Part print with two shaded views. Sizes in mm from the minimum x, y, z corner. A direction names the side the tool comes from. Give positions to 0.01 mm unless a question says otherwise; leave off trailing zeros. Write each loop counter-clockwise with the first axis right and the second up, starting at its lowest first coordinate (ties: lowest second). Pieces come first, ordered by that corner, then holes. Notation, with made-up numbers: (-20, 23.25) -> (11, 23.25) arc R25 ccw to (11, 60.25) -> close; hole circle Ø5 at (-11, -7.5). An arc over 180 degrees is marked (long way). Answer in a Markdown table with one row per item. Add a question column.
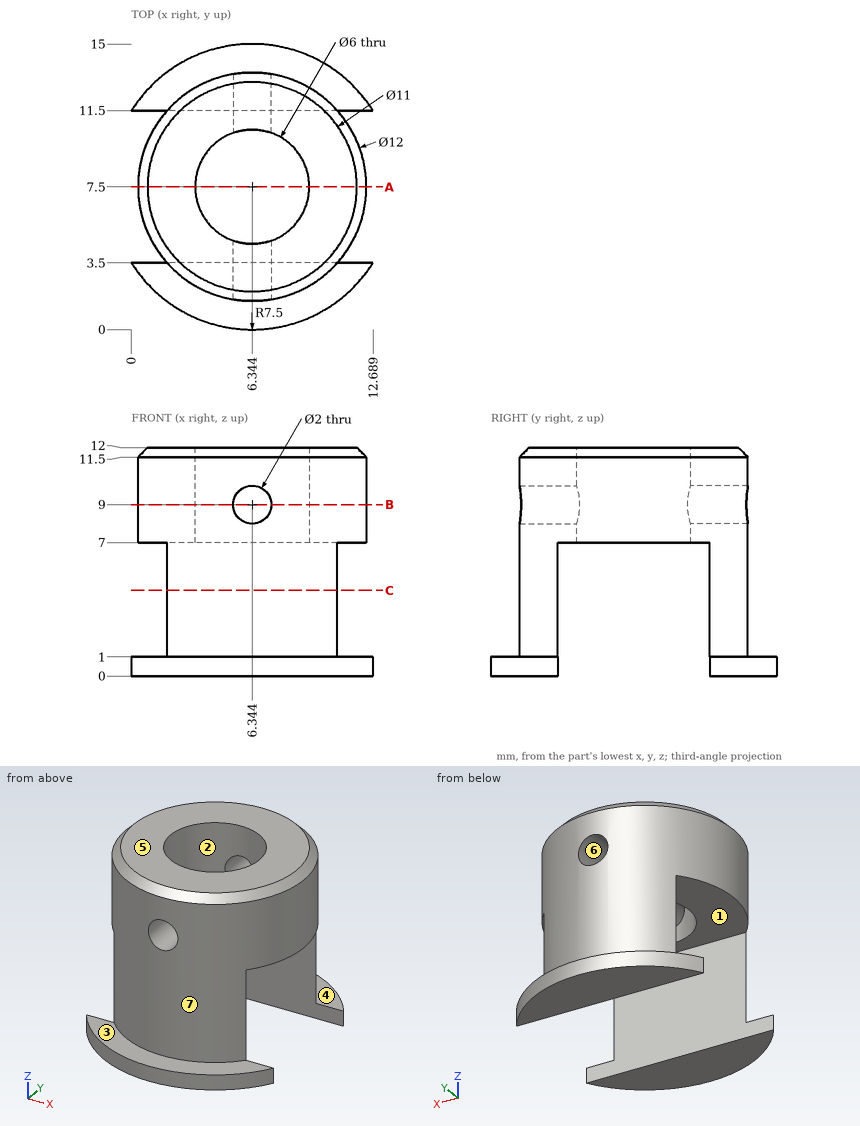
Item 1: Slice it at B-B, the plane z = 9. List the corners of the cut face in (x, y) (1 decimal).
Item 2: Slice it at C-C, the plane z = 4.5. List the corners of the cut face in (x, y) (1 decimal).
Item 3: Drop flat-ended pins along their axis: pin 1 Ø3 at (x, y) = (2, 12.5) entering from -Z; pin 2 Ø3 at (x, z) = (9, 3) entering from +Y; pin 3 Ø2 at (x, z) = (6.5, 4.5) entering from -Y. Give the stop position or say it passes through.
Item 4: Mould opens along X. For the marked faces 5, 6 and 7 say: released by +X, released by -X, zero draft, split by the parting line, or undercut.
Item 5: Slice it at A-A, the plane y = 7.5. List the corners of the cut face in (x, z) (1 decimal).
Item 6: Probe L1, parallel to Z at x = 9.5, y = 2; L2, parallel to Z at x = 2.25, y = 9.5; L3, parallel to Y at x = 3.75, z = 11.25 (1 decimal). List the from-to ranges inside material, lowest first. Write a range as from..to.
Item 7: Which spindle directions (+Z, -Z, +X, -X, +Y, -Y) get a long thin tool onto all of the face, cutting with end or side? Do the marked faces 1, 2, 3 and 4. Say none if no direction does.
Answer key:
| question | item | result |
|---|---|---|
| 1 | outline | (5.3, 1.6) -> (5.3, 4.7) arc R3 cw to (5.3, 10.3) -> (5.3, 13.4) arc R6 ccw to start; (7.3, 1.6) arc R6 ccw to (7.3, 13.4) -> (7.3, 10.3) arc R3 cw to (7.3, 4.7) -> close |
| 2 | outline | (1.9, 3.5) arc R6 ccw to (10.8, 3.5) -> close; (1.9, 11.5) -> (10.8, 11.5) arc R6 ccw to start |
| 3 | pin 1 | stops at z = 0 |
| 3 | pin 2 | stops at y = 13.39 |
| 3 | pin 3 | stops at y = 1.5 |
| 4 | face 5 | zero draft |
| 4 | face 6 | undercut |
| 4 | face 7 | split by the parting line |
| 5 | outline | (0.3, 7) -> (3.3, 7) -> (3.3, 12) -> (0.8, 12) -> (0.3, 11.5) -> close; (9.3, 7) -> (12.3, 7) -> (12.3, 11.5) -> (11.8, 12) -> (9.3, 12) -> close |
| 6 | L1 | z = 0..1 |
| 6 | L2 | z = 7..12 |
| 6 | L3 | y = 2.1..6, 9..12.9 |
| 7 | face 1 | -Z, +X, -X |
| 7 | face 2 | +Z, -Z |
| 7 | face 3 | +Z, -Y |
| 7 | face 4 | +Z, +Y |
